Autodesk Inventor part; units mm, degrees
ref_plane "YZ Plane" through (0, 0, 0) normal (1, 0, 0) x (0, 1, 0)
ref_plane "XZ Plane" through (0, 0, 0) normal (0, 1, 0) x (-1, 0, 0)
ref_plane "XY Plane" through (0, 0, 0) normal (0, 0, 1) x (1, 0, 0)
sketch "スケッチ1" plane through (0, 0, 0) normal (0, 0, 1) x (1, 0, 0)
  line L0 (0, 0) -> (15, 0)
  line L1 (15, 0) -> (15, 15)
  line L2 (15, 15) -> (0, 15)
  line L3 (0, 15) -> (0, 0)
  dimension "d0" = 15
  dimension "d1" = 15
extrude "押し出し1" add sketch "スケッチ1" along normal blind 150
sketch "スケッチ2" plane through (0, 0, 0) normal (0, 0, -1) x (-1, 0, 0)
  line L0 (0, 0) -> (-15, 0)
  line L1 (-15, 0) -> (-15, 15)
  line L2 (-15, 15) -> (0, 15)
  line L3 (0, 15) -> (0, 0)
  dimension "d4" = 15
  dimension "d5" = 15
extrude "押し出し2" cut sketch "スケッチ2" against normal blind 30
sketch "スケッチ4" plane through (0, 0, 30) normal (0, 0, -1) x (-1, 0, 0)
  line L0 (0, 0) -> (-15, 0)
  line L1 (-15, 15) -> (0, 15)
  line L2 (0, 0) -> (-15, 0)
  line L3 (-15, 0) -> (-15, 15)
  line L4 (-15, 15) -> (0, 15)
  line L5 (0, 15) -> (0, 0)
  dimension "d8" = 15
  dimension "d9" = 15
extrude "押し出し3" add sketch "スケッチ4" along normal blind 15
sketch "スケッチ5" plane through (0, 0, 150) normal (0, 0, 1) x (1, 0, 0)
  line L0 (0, 0) -> (15, 0)
  line L1 (15, 0) -> (15, 15)
  line L2 (15, 15) -> (0, 15)
  line L3 (0, 15) -> (0, 0)
  dimension "d14" = 15
  dimension "d15" = 15
extrude "押し出し4" add sketch "スケッチ5" along normal blind 15
sketch "スケッチ6" plane through (0, 0, 15) normal (0, 0, -1) x (-1, 0, 0)
  line L0 (-15, 0) -> (0, 0)
  line L1 (0, 0) -> (-15, 0)
  line L2 (-15, 0) -> (-15, 15)
  line L3 (-15, 15) -> (0, 15)
  line L4 (0, 15) -> (0, 0)
  dimension "d18" = 15
  dimension "d19" = 15
extrude "押し出し5" add sketch "スケッチ6" along normal blind 55
sketch "スケッチ7" plane through (0, 0, -40) normal (0, 0, -1) x (-1, 0, 0)
  line L0 (0, 0) -> (-15, 0)
  line L1 (-15, 0) -> (-15, 15)
  line L2 (-15, 15) -> (0, 15)
  line L3 (0, 15) -> (0, 0)
  dimension "d22" = 15
  dimension "d23" = 15
extrude "押し出し6" add sketch "スケッチ7" along normal blind 3
sketch "スケッチ8" plane through (0, 0, -43) normal (0, 0, -1) x (-1, 0, 0)
  line L0 (0, 0) -> (-15, 0)
  line L1 (-15, 0) -> (-15, 15)
  line L2 (-15, 15) -> (0, 15)
  line L3 (0, 15) -> (0, 0)
  dimension "d26" = 15
  dimension "d27" = 15
extrude "押し出し7" add sketch "スケッチ8" along normal blind 2
sketch "スケッチ9" plane through (0, 15, 165) normal (0, 1, 0) x (1, 0, 0)
  circle A0 centre (7.5, 142.5) radius 1.6
  line L0 (0, 210) -> (15, 210)
  line L1 (0, 210) -> (0, 0)
  point P0 (0, 165)
  dimension "d30" = 3.2
  dimension "d31" = 67.5
  dimension "d32" = 7.5
hole "穴1" at (7.5, 15, 22.5) direction (0, -1, 0) diameter 3.2 end through all
sketch "スケッチ10" plane through (0, 0, -45) normal (0, 0, -1) x (-1, 0, 0)
  line L0 (0, 0) -> (-15, 0)
  line L1 (-15, 0) -> (-15, 15)
  line L2 (-15, 15) -> (0, 15)
  line L3 (0, 15) -> (0, 0)
extrude "押し出し8" add sketch "スケッチ10" along normal blind 15
sketch "スケッチ11" plane through (0, 15, 165) normal (0, 1, 0) x (1, 0, 0)
  line L0 (0, 225) -> (15, 225)
  line L1 (0, 225) -> (0, 0)
  point P0 (0, 165)
  point P1 (7.5, 215)
  point P2 (7.5, 205)
  point P3 (7.5, 195)
  dimension "d42" = 10
  dimension "d43" = 7.5
  dimension "d44" = 10
  dimension "d45" = 10
hole "穴2" at (7.5, 15, -50) at (7.5, 15, -40) at (7.5, 15, -30) direction (0, -1, 0) diameter 3.2 end through all
sketch "スケッチ12" plane through (15, 0, 165) normal (1, 0, 0) x (0, 0, -1)
  point P0 (165, 0)
sketch "スケッチ13" plane through (0, 15, 165) normal (0, 1, 0) x (1, 0, 0)
  line L0 (0, 225) -> (0, 0)
  line L1 (15, 0) -> (0, 0)
  line L2 (15, 225) -> (15, 0)
  point P0 (0, 165)
  point P1 (7.5, 10)
  point P2 (7.5, 20)
  point P3 (7.5, 30)
  dimension "d53" = 7.5
  dimension "d54" = 10
  dimension "d55" = 10
  dimension "d56" = 10
  dimension "d57" = 7.5
  dimension "d58" = 7.5
hole "穴3" at (7.5, 15, 155) at (7.5, 15, 145) at (7.5, 15, 135) direction (0, -1, 0) diameter 3.2 end through all
sketch "スケッチ14" plane through (0, 15, 165) normal (0, 1, 0) x (1, 0, 0)
  circle A0 centre (7.5, 142.5) radius 1.6
  line L0 (0, 225) -> (0, 0)
  line L1 (15, 225) -> (15, 0)
  point P0 (0, 165)
  point P1 (7.5, 152.5)
  point P2 (7.5, 132.5)
  dimension "d66" = 10
  dimension "d67" = 7.5
  dimension "d68" = 10
  dimension "d69" = 7.5
hole "穴4" at (7.5, 15, 32.5) at (7.5, 15, 12.5) direction (0, -1, 0) diameter 3.2 end through all
sketch "スケッチ15" plane through (0, 0, 165) normal (0, 0, 1) x (1, 0, 0)
  line L0 (1.5, 1.5) -> (13.5, 1.5)
  line L1 (13.5, 1.5) -> (13.5, 13.5)
  line L2 (13.5, 13.5) -> (1.5, 13.5)
  line L3 (1.5, 13.5) -> (1.5, 1.5)
  line L4 (0, 0) -> (15, 0)
  line L5 (0, 15) -> (0, 0)
  dimension "d77" = 12
  dimension "d78" = 12
  dimension "d79" = 1.5
  dimension "d80" = 1.5
extrude "押し出し9" cut sketch "スケッチ15" against normal blind 1400
sketch "スケッチ16" plane through (15, 0, 165) normal (1, 0, 0) x (0, 0, -1)
  line L0 (225, 15) -> (0, 15)
  line L1 (225, 15) -> (225, 0)
  line L2 (0, 0) -> (0, 15)
  line L3 (225, 0) -> (0, 0)
  point P0 (165, 0)
  point P1 (175, 7.5)
  point P2 (50, 7.5)
  point P3 (0, 7.5)
  dimension "d83" = 7.5
  dimension "d84" = 50
  dimension "d85" = 50
  dimension "d86" = 7.5
hole "穴5" at (15, 7.5, 115) at (15, 7.5, -10) direction (-1, 0, 0) diameter 3.2 end through all
properties part number "射出_角柱3" material "アルミニウム 6061"
Source: CAD feature listing. Evaluate the final solid. Frame: model axes, mm. A direction names the side the tool comes from. Give positions to 0.01 mm unless a question says otherwise; leave off trailing zeros. Write each loop counter-clockwise with the first axis right and the second up, starting at its lowest first coordinate (ties: lowest second). Pieces come first, ordered by that corner, then holes. Notation, with made-up numbers: (29, -34.75) -> (42, -34.75) arc R23 cw to (42, -10.75) -> close; hole circle Ø10 at (20.25, 76.25). An arc over 180 degrees is marked (long way). Write item = value, one per line.
Q1. Mould query, pull axis Y, two halves, no side actions, for faces 1 (the face through (8, 15, 54)), 2 (the face through (1.5, 8, 54)), 3 (the face through (0, 8, 54)). Classes: +Y half, -Y half, draft (parallel to the pull), parting line (faces both ways), or undercut.
Here are the results:
face_1 = +Y half
face_2 = undercut
face_3 = draft
Q2. Cut plane A-A on z = 66. Return loops of the section in (x, y), then the cut area to 3 significant figures.
Here are the results:
outline = (0, 0) -> (15, 0) -> (15, 15) -> (0, 15) -> close; hole (1.5, 1.5) -> (13.5, 1.5) -> (13.5, 13.5) -> (1.5, 13.5) -> close
area = 81.0 mm²
Q3. First-contact query: pin 1 (3 mm diameter, centred on x = 7.5, z = 22.5, fed in from -Y). Flat tip, straight axial feed; report the tip coordinate or a pass-through.
Here are the results:
pin_1 = through
Q4. Reachability of faces 4 (the face through (13.5, 7, 54)), 5 (the face through (1, 8, -60)) from +Z, -Z, +X, -X, +Y, -Y: full face, straight path, thin tool, end or side. Return the list, or none.
Here are the results:
face_4 = +Z, -Z
face_5 = -Z, +X, -X, +Y, -Y
Q5. Line query: line 1 (Z direction, x = 0.9, y = 7.5); line 2 (Y direction, x = 8.75, z = 69.5). Output: solid intervals per line, ascending. Write a range as from..to.
Here are the results:
line_1 = -60..-11.6, -8.4..113.4, 116.6..165
line_2 = 0..1.5, 13.5..15
Q6. Cut plane B-B on y = 3.5. Return loops of the section in (x, z).
Here are the results:
outline = (0, -60) -> (1.5, -60) -> (1.5, 165) -> (0, 165) -> close; (13.5, -60) -> (15, -60) -> (15, 165) -> (13.5, 165) -> close
